```python
from build123d import *

# Parameters (mm, degrees)
SKETCH1_R           = 100
BOSS_EXTRUDE1_DEPTH = 50
SKETCH2_W           = 300
SKETCH2_H           = 75
BOSS_EXTRUDE2_DEPTH = 50
SKETCH3_R           = 10
SKETCH3_R_2         = 15
BOSS_EXTRUDE3_DEPTH = 37.5
SKETCH4_W           = 75
SKETCH4_H           = 72.5
SKETCH4_W_2         = 50
SKETCH4_H_2         = 55
CUT_EXTRUDE2_DEPTH  = 25
CHAMFER1_SIZE       = 10
CHAMFER2_SIZE       = 10


with BuildPart() as part:
    # Sketch1 → Boss-Extrude1 (new body)
    with BuildSketch(Plane(origin=(0, 0, 0), x_dir=(1, 0, 0), z_dir=(0, 1, 0))):
        with Locations(Location((0, 0, 0), (0, 0, 270))):
            Circle(SKETCH1_R)
    extrude(amount=BOSS_EXTRUDE1_DEPTH)

    # Sketch2 → Boss-Extrude2 (add)
    with BuildSketch(Plane(origin=(0, 50, 0), x_dir=(1, 0, 0), z_dir=(0, 1, 0))):
        with Locations((-150, 0)):
            Rectangle(SKETCH2_W, SKETCH2_H)
    extrude(amount=-BOSS_EXTRUDE2_DEPTH)

    # Sketch3 → Boss-Extrude3 (add, symmetric)
    # profile 1 of 2: a face of its own
    with BuildSketch(Plane.XY):
        with BuildLine():
            Line((-300, 50), (-300, 80))
            ThreePointArc((-300, 80), (-275, 105), (-250, 80))
            Line((-250, 80), (-250, 50))
            Line((-250, 50), (-300, 50))
        make_face()
        with Locations((-275, 80)):
            Circle(SKETCH3_R, mode=Mode.SUBTRACT)
    # profile 2 of 2: a face of its own
    with BuildSketch(Plane.XY):
        with BuildLine():
            Line((-37.5, 50), (37.5, 50))
            Line((37.5, 50), (37.5, 250))
            ThreePointArc((37.5, 250), (0, 287.5), (-37.5, 250))
            Line((-37.5, 250), (-37.5, 50))
        make_face()
        with Locations((0, 250)):
            Circle(SKETCH3_R_2, mode=Mode.SUBTRACT)
    extrude(amount=BOSS_EXTRUDE3_DEPTH, both=True)

    # Sketch4 → Cut-Extrude2 (cut, symmetric)
    with BuildSketch(Plane.XY):
        with Locations((0, 251.25)):
            Rectangle(SKETCH4_W, SKETCH4_H)
        with Locations((-275, 77.5)):
            Rectangle(SKETCH4_W_2, SKETCH4_H_2)
    extrude(amount=CUT_EXTRUDE2_DEPTH, both=True, mode=Mode.SUBTRACT)

    # Chamfer1
    chamfer1_edges = [part.edges().sort_by_distance(p)[0] for p in [
        (-171.351240544, 50, -37.5),
        (100, 50, 0),
        (-171.351240544, 50, 37.5),
    ]]
    chamfer(chamfer1_edges, length=CHAMFER1_SIZE)

    # Chamfer2
    chamfer2_edges = [part.edges().sort_by_distance(p)[0] for p in [
        (0, 50, 37.5),
        (0, 50, -37.5),
        (-37.5, 50, 0),
        (37.5, 50, 0),
    ]]
    chamfer(chamfer2_edges, length=CHAMFER2_SIZE)


solid = part.part
```
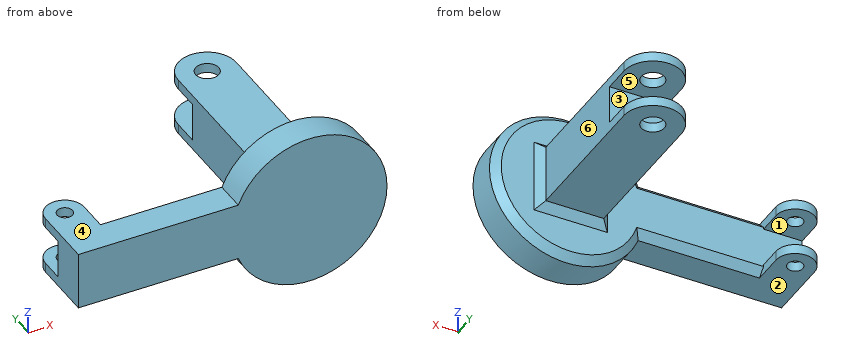
CAD build for the part. Positions are in the model's coordinates, mm. Face numbers are marked on the shaded views. A direction names the side the tool comes from. Round coordinates to 2 decimals unless told otherwise and drop trailing zeros. Write each loop counter-clockwise with the first axis right and the second up, starting at its lowest first coordinate (ties: lowest second). Pieces come first, ordered by that corner, then holes. Notation, with made-up numbers: (33, -0.5) -> (60, -0.5) arc R35 ccw to (60, 38.5) -> close; hole circle Ø8 at (51.25, 45.25). An arc over 180 degrees is marked (long way). Answer in a Markdown table with one row per item. Add a question column.
Item 1: Drill centre lines: line 1 (X direction, y = 80, z = 28); line 2 (Y direction, x = -275, z = -32.25); line 3 (Y direction, x = 0, z = -33). Where is each one in solid material? Low to high. Write a range as from..to.
Item 2: Mould opens along Z. For the marked faces 4, 5 and 6 say: pulls with the +Z half, pulls with the -Z half, needs draft (parallel to the pull), parting line crosses it, or undercut.
Item 3: Saw through at B-B, the plane z = 0. Write the cut outline in (x, y), then the cut area to 3 significant figures.
Item 4: Saw through at C-C, the plane x = 0. Write the cut outline in (y, z).
Item 5: Saw through at A-A, the plane x = -275. Write the cut outline in (y, z).
Item 6: Drop flat-ended pins along their axis: pin 1 Ø12 at (x, z) = (16.5, 11) entering from -Y; pin 2 Ø22.5 at (x, y) = (-11.5, 190) entering from -Z; pin 3 Ø1.5 at (x, z) = (-203.5, -32.5) entering from +Y; pin 4 Ø1 at (y, z) = (63, -32.5) entering from +X. Give the stop position or say it passes through.
Item 7: Which spindle directions (+Z, -Z, +X, -X, +Y, -Y) get a long thin tool onto all of the face, cutting with end or side? Do the marked faces 1, 2 and 3. Say none if no direction does.
Item 8: Saw through at D-D, the plane y = 122. Write the cut outline in (x, z).
Findings below:
| question | item | result |
|---|---|---|
| 1 | line 1 | x = -300..-285, -265..-250, -37.5..37.5 |
| 1 | line 2 | y = 0..70, 90..105 |
| 1 | line 3 | y = 0..235, 265..287.5 |
| 2 | face 4 | pulls with the +Z half |
| 2 | face 5 | undercut |
| 2 | face 6 | needs draft |
| 3 | outline | (-300, 0) -> (100, 0) -> (100, 40) -> (90, 50) -> (47.5, 50) -> (37.5, 60) -> (37.5, 215) -> (-37.5, 215) -> (-37.5, 60) -> (-47.5, 50) -> (-300, 50) -> close |
| 3 | area | 32,400 mm^2 |
| 4 | outline | (0, -100) -> (40, -100) -> (50, -90) -> (50, -47.5) -> (60, -37.5) -> (235, -37.5) -> (235, -25) -> (215, -25) -> (215, 25) -> (235, 25) -> (235, 37.5) -> (60, 37.5) -> (50, 47.5) -> (50, 90) -> (40, 100) -> (0, 100) -> close; (265, -37.5) -> (287.5, -37.5) -> (287.5, -25) -> (265, -25) -> close; (265, 25) -> (287.5, 25) -> (287.5, 37.5) -> (265, 37.5) -> close |
| 5 | outline | (0, -37.5) -> (70, -37.5) -> (70, -25) -> (50, -25) -> (50, 25) -> (70, 25) -> (70, 37.5) -> (0, 37.5) -> close; (90, -37.5) -> (105, -37.5) -> (105, -25) -> (90, -25) -> close; (90, 25) -> (105, 25) -> (105, 37.5) -> (90, 37.5) -> close |
| 6 | pin 1 | stops at y = 0 |
| 6 | pin 2 | stops at z = -37.5 |
| 6 | pin 3 | stops at y = 45.75 |
| 6 | pin 4 | stops at x = 37.5 |
| 7 | face 1 | -X, +Y |
| 7 | face 2 | -Z, -X, +Y, -Y |
| 7 | face 3 | +X, -X, +Y |
| 8 | outline | (-37.5, -37.5) -> (37.5, -37.5) -> (37.5, 37.5) -> (-37.5, 37.5) -> close |
